Check sheet for the modelled part. Datum: model origin and axes. Units: mm. Face numbers are marked on the shaded views. A direction names the side the tool comes from. Coordinates: 2 decimals unless noted, no trailing zeros. Loops run counter-clockwise (first coordinate to the right, second up) from the corner with the lowest first, then second, coordinate; pieces in that order, holes last. Notation, with made-up numbers: M 26,-14 L 85,-14 A28 cw 85,24 Z; hole C 17,-21 d2. An arc over 180 degrees is marked long. Use CSV: the item, a comma, the result in double quotes. Start each with the question number.
(1) Go/stop test with flat-tipped pins: pin 1 Ø7.5 at (x, y) = (15, 2.5) entering from -Z; pin 2 Ø4 at (x, z) = (26.5, 4) entering from +Y; pin 3 Ø3.5 at (x, y) = (14.5, 2) entering from +Z; pin 4 Ø8 at (x, z) = (39.5, 15.5) entering from +Y. Record where each tip stops, or that it passes through.
(2) Section check A-A on z = 14. Give the number of separate pieces and of enclosed holes in the cut face, and give its area (3 significant figures).
(3) Section check B-B on x = 43.5. Record the cut outline in (y, z), and give its area (3 significant figures).
(4) Set-up check for the marked faces 1, 2, 3 and 4: record each of +Z, -Z, +X, -X, +Y, -Y from which the full face is reachable in a straight line by a thin tool's end or side.
(5) Draft check along X on the marked faces 5, 6 and 7. Enter one of: pulls with the +X half, pulls with the -X half, needs draft (parallel to the pull), parting line crosses it, or undercut.
(6) Section check D-D on x = 15. Record the cut outline in (y, z).
(7) Section check C-C on z = 1.75. Record the cut outline in (x, y), and give its area (3 significant figures).
(8) Scan lines: line 1 (X direction, y = 1.1, z = 14); line 2 (Y direction, x = 24, z = 1.5); line 3 (X direction, y = 2.5, z = 3.25). Record each from-to range of solid material in increasing order.
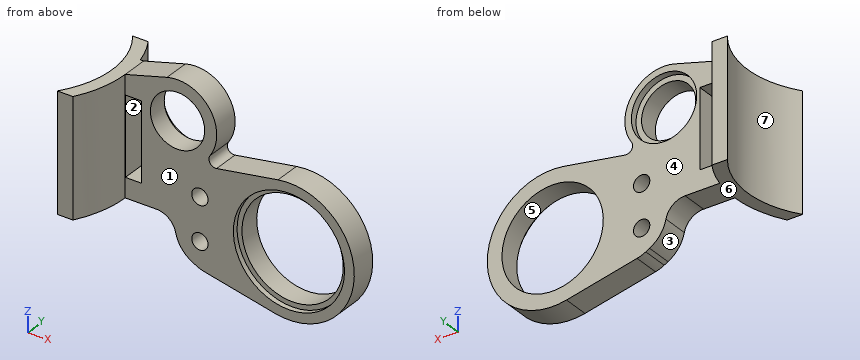
from build123d import *

# Parameters (mm, degrees)
EXTRUDE_1_DEPTH     = 18
SKETCH_3_R          = 4.15
SKETCH_3_R_2        = 7.75
SKETCH_3_R_3        = 1.25
SKETCH_3_W          = 2.5
SKETCH_3_H          = 12
EXTRUDE_2_DEPTH     = 4
FILLET_1_R          = 5
FILLET_2_R          = 3
FILLET_3_R          = 1
SKETCH_7_R          = 8.5
CUT_EXTRUDE_2_DEPTH = 0.8
SKETCH_8_R          = 5
CUT_EXTRUDE_3_DEPTH = 1


with BuildPart() as part:
    # 草图1 → 凸台-拉伸1 (new body)
    with BuildSketch(Plane.XY):
        with BuildLine():
            Line((13.754950724, 8.173208097), (11.36655926, 8.173208097))
            ThreePointArc((11.36655926, 8.173208097), (14, 0), (11.36655926, -8.173208097))
            Line((11.36655926, -8.173208097), (13.754950724, -8.173208097))
            ThreePointArc((13.754950724, -8.173208097), (16, 0), (13.754950724, 8.173208097))
        make_face()
    extrude(amount=EXTRUDE_1_DEPTH)

    # 草图3 → 凸台-拉伸2 (add)
    with BuildSketch(Plane(origin=(0, 0, 0), x_dir=(1, 0, 0), z_dir=(0, 1, 0))):
        with BuildLine():
            Line((16, -18), (14.877475362, -18))
            Line((14.877475362, -18), (14.877475362, 0))
            Line((14.877475362, 0), (16, 0))
            Line((16, 0), (23.606969391, 0))
            Line((23.606969391, 0), (23.606969391, 4.353528312))
            Line((23.606969391, 4.353528312), (27.426147231, 6.432993818))
            Line((27.426147231, 6.432993818), (38.92049676, 8.930407807))
            ThreePointArc((38.92049676, 8.930407807), (51.041058959, -0.612171869), (39.370999256, -10.700708007))
            Line((39.370999256, -10.700708007), (26.396794679, -8.499511361))
            ThreePointArc((26.396794679, -8.499511361), (29.653921129, -16.00827684), (22.389974874, -19.779949748))
            Line((22.389974874, -19.779949748), (16, -18))
        make_face()
        with Locations(Location((24, -14, 0), (0, 0, 270))):
            Circle(SKETCH_3_R, mode=Mode.SUBTRACT)
        with Locations(Location((41.043691062, -0.841595363, 0), (0, 0, 270))):
            Circle(SKETCH_3_R_2, mode=Mode.SUBTRACT)
        with Locations(Location((27.426147231, -4.091595363, 0), (0, 0, 270))):
            Circle(SKETCH_3_R_3, mode=Mode.SUBTRACT)
        with Locations(Location((27.426147231, 2.408404637, 0), (0, 0, 270))):
            Circle(SKETCH_3_R_3, mode=Mode.SUBTRACT)
        with Locations((17.267287819, -9)):
            Rectangle(SKETCH_3_W, SKETCH_3_H, mode=Mode.SUBTRACT)
    extrude(amount=EXTRUDE_2_DEPTH)

    # 圆角1
    fillet_1_edges = [part.edges().sort_by_distance(p)[0] for p in [
        (27.426147231, 2, -6.432993818),
        (23.606969391, 2, -4.353528312),
    ]]
    fillet(fillet_1_edges, radius=FILLET_1_R)

    # 圆角2
    fillet_2_edges = [part.edges().sort_by_distance(p)[0] for p in [
        (23.606969391, 2, 0),
    ]]
    fillet(fillet_2_edges, radius=FILLET_2_R)

    # 圆角3
    fillet_3_edges = [part.edges().sort_by_distance(p)[0] for p in [
        (26.396794679, 2, 8.499511361),
    ]]
    fillet(fillet_3_edges, radius=FILLET_3_R)

    # 草图7 → 切除-拉伸2 (cut)
    with BuildSketch(Plane.XZ):
        with Locations(Location((41.043691062, 0.841595363, 0), (0, 0, 270))):
            Circle(SKETCH_7_R)
    extrude(amount=-CUT_EXTRUDE_2_DEPTH, mode=Mode.SUBTRACT)

    # 草图8 → 切除-拉伸3 (cut)
    with BuildSketch(Plane(origin=(0, 4, 0), x_dir=(1, 0, 0), z_dir=(0, 1, 0))):
        with Locations(Location((24, -14, 0), (0, 0, 270))):
            Circle(SKETCH_8_R)
    extrude(amount=-CUT_EXTRUDE_3_DEPTH, mode=Mode.SUBTRACT)


solid = part.part
Outcome:
1,pin 1,"stops at z = 0"
1,pin 2,"stops at y = 4"
1,pin 3,"stops at z = 18.07"
1,pin 4,"passes through"
2,separate pieces,"3"
2,enclosed holes,"0"
2,area,"46.4 mm²"
3,outline,"M 0,-8.85 L 4,-8.85 L 4,-6.51 L 0.8,-6.51 L 0.8,-7.3 L 0,-7.3 Z; M 0,8.98 L 0.8,8.98 L 0.8,8.19 L 4,8.19 L 4,10.54 L 0,10.54 Z"
3,area,"17.5 mm²"
4,face 1,"+Z, -Z, +X, -Y"
4,face 2,"+Y, -Y"
4,face 3,"-Z, -X, +Y, -Y"
4,face 4,"+Z, -Z, +X, +Y"
5,face 5,"undercut"
5,face 6,"needs draft"
5,face 7,"pulls with the -X half"
6,outline,"M -5.57,0 L 5.57,0 L 5.57,18 L -5.57,18 Z"
7,outline,"M 11.37,-8.17 L 13.75,-8.17 A16 ccw 16,0 L 32.59,0 L 32.59,0.8 L 33.35,0.8 L 33.35,4 L 15.49,4 A16 ccw 13.75,8.17 L 11.37,8.17 A14 cw Z; M 48.74,0.8 L 49.5,0.8 L 49.5,0 L 51,0 L 51,4 L 48.74,4 Z"
7,area,"112 mm²"
8,line 1,"x = 13.96 to 16.02, 18.52 to 19.85, 28.15 to 30"
8,line 2,"y = 0 to 4"
8,line 3,"x = 13.77 to 16.02, 18.52 to 26.5, 28.35 to 33.68, 48.41 to 50.75"
